Autodesk Inventor part; units mm, degrees
ref_plane "YZ Plane" through (0, 0, 0) normal (1, 0, 0) x (0, 1, 0)
ref_plane "XZ Plane" through (0, 0, 0) normal (0, 1, 0) x (-1, 0, 0)
ref_plane "XY Plane" through (0, 0, 0) normal (0, 0, 1) x (1, 0, 0)
sketch "Sketch1" plane through (0, 0, 0) normal (0, 0, 1) x (1, 0, 0)
  line L0 (0, 0) -> (27, 0)
  line L1 (27, 0) -> (27, -4.6)
  line L2 (27, -4.6) -> (0, -4.6)
  line L3 (0, -4.6) -> (0, 0)
  circle A0 centre (2.2589, -2.3) radius 1.25
  dimension "d0" = 2.3
  dimension "d1" = 2.3
  dimension "d2" = 27
  dimension "d12" = 2.5
extrude "Extrusion1" add sketch "Sketch1" along normal blind 2
sketch "Sketch2" plane through (0, 0, 0) normal (0, 0, -1) x (-1, 0, 0)
  line L0 (0, -4.6) -> (-27, -4.6)
  line L1 (-6.3, 0) -> (-8.3, 0)
  line L2 (-8.3, 0) -> (-8.3, -4.6)
  line L3 (-8.3, -4.6) -> (-6.3, -4.6)
  line L4 (-6.3, -4.6) -> (-6.3, 0)
  line L5 (-27, 0) -> (0, 0)
  line L6 (-27, -4.6) -> (-25, -4.6)
  line L7 (-25, -4.6) -> (-25, 0)
  line L8 (-25, 0) -> (-27, 0)
  line L9 (-27, 0) -> (-27, -4.6)
  dimension "d5" = 2
  dimension "d6" = 2
  dimension "d7" = 16.7
extrude "Extrusion2" add sketch "Sketch2" along normal blind 7.3 contours L0 L2 L1 L4 | L0 L9 L5 L7
sketch "Sketch3" plane through (0, 0, -7.3) normal (0, 0, -1) x (-1, 0, 0)
  line L0 (-6.3, 0) -> (-8.3, 0)
  line L1 (-8.3, 0) -> (-8.3, -4.6)
  line L2 (-8.3, -4.6) -> (-6.3, -4.6)
  line L3 (-6.3, -4.6) -> (-6.3, 0)
  line L4 (-27, -4.6) -> (-25, -4.6)
  line L5 (-25, -4.6) -> (-25, 0)
  line L6 (-25, 0) -> (-27, 0)
  line L7 (-27, 0) -> (-27, -4.6)
  line L8 (-8.3, 0) -> (-25, 0)
  line L9 (-25, 0) -> (-25, -4.6)
  line L10 (-25, -4.6) -> (-8.3, -4.6)
  line L11 (-8.3, -4.6) -> (-8.3, 0)
  point P0 (0, 0)
extrude "Extrusion3" add sketch "Sketch3" along normal blind 2
equation "\"BendRadius\" = Thickness"
equation "\"BendReliefWidth\" = Thickness"
equation "\"BendReliefDepth\" = 0.5 * Thickness"
equation "\"CornerReliefSize\" = 4 * Thickness"
equation "\"MinimumRemnant\" = 2 * Thickness"
equation "\"TransitionRadius\" = BendRadius"
equation "\"JacobiRadiusSize\" = BendRadius"
equation "\"GapSize\" = Thickness"
properties part number "Switch_Holder"
Work out the finished part from the listing and answer in its coordinate system (mm). A direction names the side the tool comes from. Round coordinates to 2 decimals unless told otherwise and drop trailing zeros. Order: outer loops, then holes, each group sorted by start corner. A loop starts at its lowest first (then second) coordinate and runs counter-clockwise, first axis right, second up. Notation, with made-up numbers: M 38,-15 L 94,-15 A36 cw 94,21 Z; hole C -40,35 d5. An arc over 180 degrees is marked long. One line per item, written item: value.
Q1. Find section A-A on z = -5.5. Write down the section's boundary in (x, y).
Derived:
outline: M 6.3,-4.6 L 8.3,-4.6 L 8.3,0 L 6.3,0 Z; M 25,-4.6 L 27,-4.6 L 27,0 L 25,0 Z
Q2. For faces 5 (the face through (0, -2, 1)), 6 (the face through (25, -2, -4)), 7 (the face through (6.3, -2, -5)), determine the directions among +Z, -Z, +X, -X, +Y, -Y from which every point of the face is accessible in a straight line to the end or side of a thin tool.
Derived:
face 5: +Z, -Z, -X, +Y, -Y
face 6: +Y, -Y
face 7: -Z, -X, +Y, -Y
Q3. Determine the mould class of faces 1 (the face through (17, -2, -7.3)), 2 (the face through (27, -2, -4)), 3 (the face through (13, -2, 2)), 4 (the face through (2.931, -3.354, 0.986)) for opening direction X: released by +X, released by -X, zero draft, split by the parting line, or undercut.
Derived:
face 1: undercut
face 2: released by +X
face 3: zero draft
face 4: undercut
Q4. Find section B-B on y = -2.3. Write down the section's boundary in (x, z).
Derived:
outline: M 0,0 L 1.01,0 L 1.01,2 L 0,2 Z; M 3.51,0 L 6.3,0 L 6.3,-9.3 L 27,-9.3 L 27,2 L 3.51,2 Z; hole M 8.3,-7.3 L 25,-7.3 L 25,0 L 8.3,0 Z
Q5. Find section D-D on y = -3.9. Write down the section's boundary in (x, z), then the cut area to 3 significant figures.
Derived:
outline: M 0,0 L 6.3,0 L 6.3,-9.3 L 27,-9.3 L 27,2 L 0,2 Z; hole M 8.3,-7.3 L 25,-7.3 L 25,0 L 8.3,0 Z
area: 125 mm²
Q6. Straight lines are drawn through the part: line 1 (X direction, y = -0.25, z = -7.25); line 2 (Z direction, x = 21.5, y = -0.6); line 3 (Z direction, x = 5.5, y = -0.25). For each, find the intervals that lie inside material, in ascending order.
Derived:
line 1: 6.3 to 8.3, 25 to 27
line 2: -9.3 to -7.3, 0 to 2
line 3: 0 to 2
Q7. Find section C-C on x = 18.5. Write down the section's boundary in (y, z), then the cut area to 3 significant figures.
Derived:
outline: M -4.6,-9.3 L 0,-9.3 L 0,-7.3 L -4.6,-7.3 Z; M -4.6,0 L 0,0 L 0,2 L -4.6,2 Z
area: 18.4 mm²
Q8. Flat-ended cylindrical pins translate along their axes: pin 1 (2 mm diameter, centred on x = 2.26, y = -2.3, fed in from +Z); pin 2 (1.4 mm diameter, centred on y = -3.5, z = -5, fed in from -X); pin 3 (1.4 mm diameter, centred on x = 4.5, y = -1.5, fed in from -Z). Find the tip coordinate at first contact, or state that the pin passes through.
Derived:
pin 1: through
pin 2: x = 6.3
pin 3: z = 0
